```python
from build123d import *

# Parameters (mm, degrees)
SKETCH2_R               = 15
BOSS_EXTRUDE1_DEPTH     = 55
CUT_EXTRUDE1_DEPTH      = 59.949130613
CUT_EXTRUDE1_DEPTH_BACK = 59.949130613
SKETCH3_W               = 17.5
SKETCH3_H               = 5
CUT_EXTRUDE2_DEPTH      = 59.949130613
CUT_EXTRUDE2_DEPTH_BACK = 59.949130613
SKETCH6_R               = 2.5
SKETCH7_W               = 5
SKETCH7_H               = 30
BOSS_EXTRUDE2_DEPTH     = 4
BOSS_EXTRUDE3_DEPTH     = 5
CUT_EXTRUDE3_DEPTH      = 60.634302356
CUT_EXTRUDE3_DEPTH_BACK = 60.634302356
SKETCH9_R               = 2.5


with BuildPart() as part:
    # Sketch2 → Boss-Extrude1 (new body)
    with BuildSketch(Plane(origin=(0, 0, 0), x_dir=(0, 0, -1), z_dir=(1, 0, 0))):
        Circle(SKETCH2_R)
    extrude(amount=-BOSS_EXTRUDE1_DEPTH)

    # Sketch3 → Cut-Extrude1 (cut, two sides: drawn at the far end of the back side and taken through both)
    with BuildSketch(Plane(origin=(0, 0, 0), x_dir=(1, 0, 0), z_dir=(0, 1, 0)).offset(-CUT_EXTRUDE1_DEPTH_BACK)):
        with Locations((-46.25, 0)):
            Rectangle(SKETCH3_W, SKETCH3_H)
    extrude(amount=CUT_EXTRUDE1_DEPTH + CUT_EXTRUDE1_DEPTH_BACK, mode=Mode.SUBTRACT)

    # Sketch6 → Cut-Extrude2 (cut, two sides: drawn at the far end of the back side and taken through both)
    with BuildSketch(Plane.XY.offset(-CUT_EXTRUDE2_DEPTH_BACK)):
        with Locations((-50, 0)):
            Circle(SKETCH6_R)
    extrude(amount=CUT_EXTRUDE2_DEPTH + CUT_EXTRUDE2_DEPTH_BACK, mode=Mode.SUBTRACT)

    # Sketch7 → Boss-Extrude2 (add)
    with BuildSketch(Plane(origin=(0, 0, 0), x_dir=(0, 0, -1), z_dir=(1, 0, 0))):
        Rectangle(SKETCH7_W, SKETCH7_H)
    extrude(amount=BOSS_EXTRUDE2_DEPTH)

    # Sketch8 → Boss-Extrude3 (add)
    with BuildSketch(Plane.XY.offset(2.5)):
        with BuildLine():
            Line((4, 15), (4, -15))
            ThreePointArc((4, -15), (19, 0), (4, 15))
        make_face()
    extrude(amount=-BOSS_EXTRUDE3_DEPTH)

    # Sketch9 → Cut-Extrude3 (cut, two sides: drawn at the far end of the back side and taken through both)
    with BuildSketch(Plane.XY.offset(2.5).offset(-CUT_EXTRUDE3_DEPTH_BACK)):
        with Locations(Location((14, 0, 0), (0, 0, 270))):
            Circle(SKETCH9_R)
    extrude(amount=CUT_EXTRUDE3_DEPTH + CUT_EXTRUDE3_DEPTH_BACK, mode=Mode.SUBTRACT)


solid = part.part
```
Here's how the part is built. I have some questions about the finished solid (model axes, mm). A direction names the side the tool comes from. Give positions to 0.01 mm unless a question says otherwise; leave off trailing zeros. Loops run counter-clockwise (first coordinate to the right, second up) from the corner with the lowest first, then second, coordinate; pieces in that order, holes last. Notation, with made-up numbers: (-6, 54) -> (49, 54) arc R26 ccw to (49, 68) -> close; hole circle Ø10 at (24, 6.5). An arc over 180 degrees is marked (long way). Use one line per item in the form item = value. Start each with the question number.
1) Imagine slicing it at A-A (x = -50). Please give me the cut outline in (y, z), then the cut area to 3 significant figures.
2) Thinking about a two-plate mould opening in Y: for faces 1 (the face through (11.56, 0.54, -0.04)), 2 (the face through (-46, 0, -2.5)), 3 (the face through (-47.69, -0.96, -8.84)), 4 (the face through (2, 15, 0)), which applies, +Y half, -Y half, draft (parallel to the pull), parting line (faces both ways), or undercut?
3) For P1, Ø9.5, axis at x = 5.5, y = 5, coming from the +Z side; P2, Ø14, axis at x = -48, y = -4, coming from the -Z side; P3, Ø5, axis at x = -14, z = -11.5, coming from the -Y side; P4, Ø10, axis at y = 6.5, z = -9.5, coming from the +X side, each with a flat end and sliding along its axis, tell me the tip position at first contact or that it passes through.
4) Please list where these lines run through material, in increasing order: line 1 along X through (y, z) = (0, -1); line 2 along Z through (x, y) = (-43.5, 0); line 3 along X through (y, z) = (-8, 4).
5) Imagine slicing it at D-D (x = 14). Please give me the cut outline in (y, z), then the cut area to 3 significant figures.
6) Imagine slicing it at C-C (z = 12). Please give me the cut outline in (x, y), then the cut area to 3 significant figures.
7) Imagine slicing it at B-B (y = 0). Please give me the cut outline in (x, z), then the cut area to 3 significant figures.
8) Which directions (+Z, -Z, +X, -X, +Y, -Y) give clear straight access to the entire face, cutting with the end or side of a thin tool? Please do faces 5 (the face through (0, 0, 7)), 6 (the face through (7, 0, -2.5)), 7 (the face through (-46, 0, 2.5)), 8 (the face through (-47.69, -0.96, 8.66)), 9 (the face through (19, 0, 0)).
Check values:
q1.outline = (-14.79, -2.5) arc R15 ccw to (-2.5, -14.79) -> (-2.5, -2.5) -> close; (-14.79, 2.5) -> (-2.5, 2.5) -> (-2.5, 14.79) arc R15 ccw to start; (2.5, -14.79) arc R15 ccw to (14.79, -2.5) -> (2.5, -2.5) -> close; (2.5, 2.5) -> (14.79, 2.5) arc R15 ccw to (2.5, 14.79) -> close
q1.area = 433 mm^2
q2.face_1 = undercut
q2.face_2 = draft
q2.face_3 = undercut
q2.face_4 = +Y half
q3.P1 = 2.5
q3.P2 = -15
q3.P3 = -12
q3.P4 = 0
q4.line_1 = -37.5 to 11.5, 16.5 to 19
q4.line_2 = -15 to -2.5, 2.5 to 15
q4.line_3 = -55 to 0
q5.outline = (-11.18, -2.5) -> (-2.5, -2.5) -> (-2.5, 2.5) -> (-11.18, 2.5) -> close; (2.5, -2.5) -> (11.18, -2.5) -> (11.18, 2.5) -> (2.5, 2.5) -> close
q5.area = 86.8 mm^2
q6.outline = (-55, -9) -> (0, -9) -> (0, 9) -> (-55, 9) -> close; hole circle Ø5 at (-50, 0)
q6.area = 970 mm^2
q7.outline = (-55, -15) -> (-52.5, -15) -> (-52.5, -2.5) -> (-55, -2.5) -> close; (-55, 2.5) -> (-52.5, 2.5) -> (-52.5, 15) -> (-55, 15) -> close; (-47.5, -15) -> (0, -15) -> (0, -2.5) -> (11.5, -2.5) -> (11.5, 2.5) -> (0, 2.5) -> (0, 15) -> (-47.5, 15) -> (-47.5, 2.5) -> (-37.5, 2.5) -> (-37.5, -2.5) -> (-47.5, -2.5) -> close; (16.5, -2.5) -> (19, -2.5) -> (19, 2.5) -> (16.5, 2.5) -> close
q7.area = 1,510 mm^2
q8.face_5 = +Z, +X, +Y, -Y
q8.face_6 = -Z, +X, +Y, -Y
q8.face_7 = -X, +Y, -Y
q8.face_8 = +Z, -Z
q8.face_9 = +Z, -Z, +X
